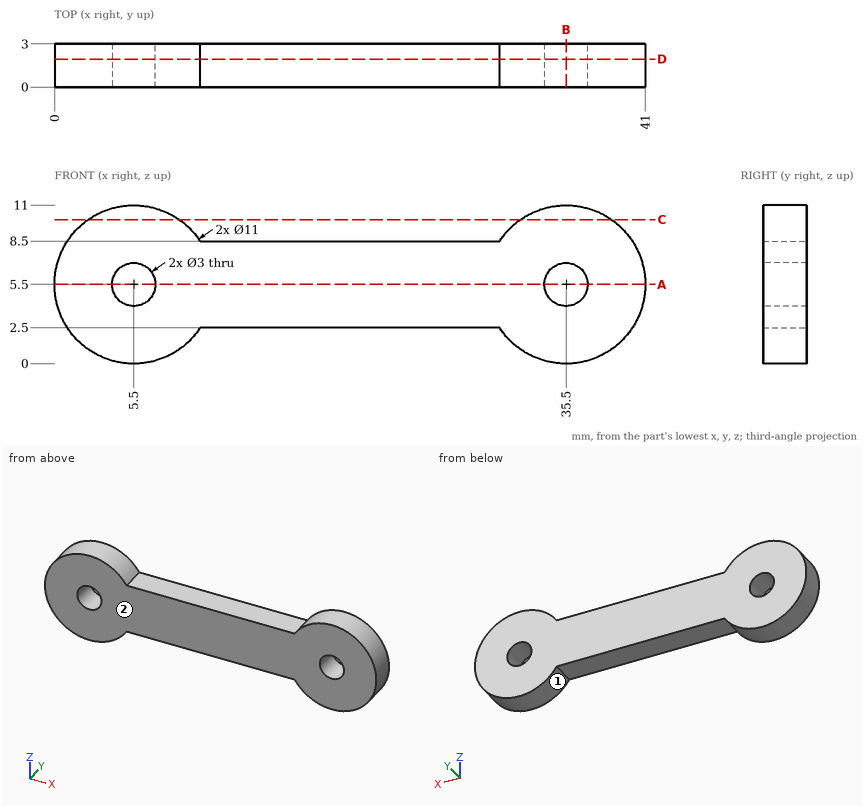
Design review of the part shown in the three views and the two pictorial views. Dimensions are in mm from the part's minimum x, y and z. Round coordinates to 2 decimals unless told otherwise and drop trailing zeros. Write each loop counter-clockwise with the first axis right and the second up, starting at its lowest first coordinate (ties: lowest second). Pieces come first, ordered by that corner, then holes.
Item 1: Consider section D-D on y = 1.95. Give the boundary of the cut face in (x, z).
Item 2: Consider section C-C on z = 10. Give the boundary of the cut face in (x, y), and give its area (3 significant figures).
Item 3: Wall thickness on L1, parallel to Z at x = 35.5, y = 0.85; L2, parallel to Z at x = 13.5, y = 0.2; L3, parallel to X at y = 1.9, z = 1.5: over which ranges is each line inside the solid? List them lowest first.
Item 4: Consider section B-B on x = 35.5. Give the boundary of the cut face in (y, z).
Item 5: For pin 1 Ø1.5 at (y, z) = (2.5, 1.5) entering from -X; pin 2 Ø1.5 at (x, y) = (25, 1.5) entering from -Z; pin 3 Ø1.5 at (x, y) = (22.5, 1.5) entering from +Z; pin 4 Ø4 at (x, z) = (5.5, 5.5) entering from +Y, all flat-tipped, find the tip position at first contact; note any pin that passes through.
Item 6: Draft analysis for pull direction X (two halves, no side actions). For the marked faces 1 and 2, state which applies: released by +X, released by -X, zero draft, split by the parting line, or undercut.
Item 7: Consider section A-A on z = 5.5. Give the boundary of the cut face in (x, y), and give its area (3 significant figures).
Check values:
1. outline: (10.11, 2.5) - (30.89, 2.5) arc R5.5 ccw (long way) to (30.89, 8.5) - (10.11, 8.5) arc R5.5 ccw (long way) to start; hole circle Ø3 at (5.5, 5.5); hole circle Ø3 at (35.5, 5.5)
2. outline: (2.34, 0) - (8.66, 0) - (8.66, 3) - (2.34, 3) - close; (32.34, 0) - (38.66, 0) - (38.66, 3) - (32.34, 3) - close
2. area: 37.9 mm2
3. L1: z = 0 to 4, 7 to 11
3. L2: z = 2.5 to 8.5
3. L3: x = 1.73 to 9.27, 31.73 to 39.27
4. outline: (0, 0) - (3, 0) - (3, 4) - (0, 4) - close; (0, 7) - (3, 7) - (3, 11) - (0, 11) - close
5. pin 1: stops at x = 1.06
5. pin 2: stops at z = 2.5
5. pin 3: stops at z = 8.5
5. pin 4: stops at y = 3
6. face 1: undercut
6. face 2: zero draft
7. outline: (0, 0) - (4, 0) - (4, 3) - (0, 3) - close; (7, 0) - (34, 0) - (34, 3) - (7, 3) - close; (37, 0) - (41, 0) - (41, 3) - (37, 3) - close
7. area: 105 mm2
